CAD build for the part. Positions are in the model's coordinates, mm. A direction names the side the tool comes from. Round coordinates to 2 decimals unless told otherwise and drop trailing zeros. Write each loop counter-clockwise with the first axis right and the second up, starting at its lowest first coordinate (ties: lowest second). Pieces come first, ordered by that corner, then holes. Notation, with made-up numbers: (-23, -14) - (6, -14) arc R9 ccw to (6, -8) - close; hole circle Ø6 at (1.25, 18.25). An arc over 180 degrees is marked (long way). Answer in a Markdown table with one row per item.
```python
from build123d import *

# Parameters (mm, degrees)
SKETCH004_W   = 36.161861
SKETCH004_H   = 4.748486
PAD002_DEPTH  = 100
PAD001_DEPTH  = 50
ARRAY_Y_COUNT = 7
ARRAY_Y_PITCH = 10
SKETCH_R      = 1.75
PAD_DEPTH     = 9
FILLET_R      = 1
FILLET002_R   = 3
FILLET003_R   = 2


with BuildPart() as pad002:
    # Sketch004 → Pad002 (new body)
    with BuildSketch(Plane(origin=(1, -50, 0), x_dir=(1, 0, 0), z_dir=(0, -1, 0))):
        with Locations((0.005565, 6.850441)):
            Rectangle(SKETCH004_W, SKETCH004_H)
    extrude(amount=-PAD002_DEPTH)


with BuildPart() as array:
    # Sketch003 → Pad001 (new body)
    with BuildSketch(Plane(origin=(-23.0697, 0, 0), x_dir=(0, -1, 0), z_dir=(-1, 0, 0))):
        with BuildLine():
            Line((-1.127729, 2.982091), (2.228669, 6.982091))
            ThreePointArc((3.377736, 6.017909), (3.285293, 7.074533), (2.228669, 6.982091))
            Line((0.021337, 2.017909), (3.377736, 6.017909))
            ThreePointArc((-1.127729, 2.982091), (-1.035287, 1.925467), (0.021337, 2.017909))
        make_face()
    extrude(amount=-PAD001_DEPTH)

    # Array Y: Array ×7


with BuildPart() as array_1:
    add(array.part)
    with Locations(*[(0, i * ARRAY_Y_PITCH, 0) for i in range(1, ARRAY_Y_COUNT)]):
        add(array.part)


with BuildPart() as array_2:
    # Array placement: moved
    add(array_1.part.moved(Location((0, -29.5, 0))))


with BuildPart() as fillet003:
    # Sketch → Pad (new body)
    with BuildSketch(Plane.XY):
        Polygon((-12.0697, 41.4218), (13.9303, 41.4218), (24.322605, 47.4218), (29.822605, 37.895521), (24.9303, 35.070947), (24.9303, -36.227347), (29.822605, -39.051921), (24.322605, -48.5782), (13.9303, -42.5782), (-12.0697, -42.5782), (-22.462005, -48.5782), (-27.962005, -39.051921), (-23.0697, -36.227347), (-23.0697, 35.070947), (-27.962005, 37.895521), (-22.462005, 47.4218), align=None)
        with Locations((-20.37566, -40.791855)):
            Circle(SKETCH_R, mode=Mode.SUBTRACT)
        with Locations((22.23626, -40.791855)):
            Circle(SKETCH_R, mode=Mode.SUBTRACT)
        with Locations((22.23626, 39.635455)):
            Circle(SKETCH_R, mode=Mode.SUBTRACT)
        with Locations((-20.37566, 39.635455)):
            Circle(SKETCH_R, mode=Mode.SUBTRACT)
        Polygon((22.9303, 35.070947), (22.9303, -36.227347), (17.35405, -40.5782), (-15.49345, -40.5782), (-21.0697, -36.227347), (-21.0697, 35.070947), (-15.49345, 39.4218), (17.35405, 39.4218), align=None, mode=Mode.SUBTRACT)
    extrude(amount=PAD_DEPTH)

    # Fillet
    fillet_edges = [fillet003.edges().sort_by_distance(p)[0] for p in [
        (-22.462005, 47.4218, 4.5),
        (24.322605, 47.4218, 4.5),
        (29.822605, 37.895521, 4.5),
        (29.822605, -39.051921, 4.5),
        (24.322605, -48.5782, 4.5),
        (-22.462005, -48.5782, 4.5),
        (-27.962005, -39.051921, 4.5),
        (-27.962005, 37.895521, 4.5),
    ]]
    fillet(fillet_edges, radius=FILLET_R)

    # Cut: cut Array
    add(array_2.part, mode=Mode.SUBTRACT)

    # Cut001: cut Pad002
    add(pad002.part, mode=Mode.SUBTRACT)

    # Fillet002
    fillet002_edges = [fillet003.edges().sort_by_distance(p)[0] for p in [
        (-17.075366, -39.343915, 6.738099),
        (-17.075366, -45.468223, 6.738099),
        (19.086495, -45.555131, 6.738099),
        (19.086495, -39.226465, 6.738099),
        (-17.075366, 44.311823, 6.738099),
        (-17.075366, 38.187515, 6.738099),
        (19.086495, 44.398731, 6.738099),
        (19.086495, 38.070065, 6.738099),
    ]]
    fillet(fillet002_edges, radius=FILLET002_R)

    # Fillet003
    fillet003_edges = [fillet003.edges().sort_by_distance(p)[0] for p in [
        (-12.0697, -42.5782, 2.238099),
        (13.9303, -42.5782, 2.238099),
        (-12.0697, 41.4218, 2.238099),
        (13.9303, 41.4218, 2.238099),
    ]]
    fillet(fillet003_edges, radius=FILLET003_R)


solid = fillet003.part
```
Q1. Drill centre lines: line 1 (X direction, y = -3.5, z = 0.5); line 2 (Y direction, x = -11, z = 3.75); line 3 (Y direction, x = 26.5, z = 1.75). Where is each one in solid material? Low to high.
Computed:
| item | result |
|---|---|
| line 1 | x = -23.07 to -21.07, 22.93 to 24.93 |
| line 2 | y = -42.58 to -40.58, 39.42 to 41.42 |
| line 3 | y = -44.81 to -37.13, 35.98 to 43.65 |
Q2. 3-axis set-ups, long thin cutter, end or side, ignore diameter. For faces 3 (the flat face through (-22.084, -1.176, 3.99)), 4 (the flat face through (-25.055, 36.217, 4.437)), 5 (the flat face through (24.93, -0.1, 5.4)): which of +Z, -Z, +X, -X, +Y, -Y reach the whole face in a straight line?
Computed:
| item | result |
|---|---|
| face 3 | +X, -X |
| face 4 | +Z, -Z, -X |
| face 5 | +Z, -Z, +X |
Q3. Saw through at A-A on x = 0. List the corners of the cut face in (y, z), then the cut area to 3 significant figures.
Computed:
| item | result |
|---|---|
| outline | (-42.58, 0) - (-40.58, 0) - (-40.58, 4.48) - (-42.58, 4.48) - close; (39.42, 0) - (41.42, 0) - (41.42, 4.48) - (39.42, 4.48) - close |
| area | 17.9 mm2 |
Q4. Flat gauge pins, fed straight in: pin 1 (1.5 mm diameter, centred on y = -41.5, z = 8, fed in from +X); pin 2 (3 mm diameter, centred on y = 41, z = 8, fed in from +X); pin 3 (3.5 mm diameter, centred on x = 2, z = 2.5, fed in from -Y); pin 4 (2.5 mm diameter, centred on x = 10, y = 43, fed in from +Z). Where does each tip first touch, or does it go through?
Computed:
| item | result |
|---|---|
| pin 1 | stops at x = 28.84 |
| pin 2 | stops at x = 28.9 |
| pin 3 | stops at y = -42.58 |
| pin 4 | passes through |
Q5. Pull direction Z, two halves, no side cores. Call faces 1 (the flat face through (-25.244, 42.604, 4.437)), 2 (the flat face through (23.916, -11.176, 3.99)): released by +Z, released by -Z, zero draft, split by the parting line, or undercut.
Computed:
| item | result |
|---|---|
| face 1 | zero draft |
| face 2 | undercut |
